Can you work these out from the model? Positions are in its coordinate system, mm. A direction names the side the tool comes from. Coordinates: 2 decimals unless noted, no trailing zeros. Order: outer loops, then holes, each group sorted by start corner. A loop starts at its lowest first (then second) coordinate and runs counter-clockwise, first axis right, second up.
```python
from build123d import *

# Parameters (mm, degrees)
SKETCH1_W           = 76.2
SKETCH1_H           = 25.4
SKETCH1_W_2         = 69.85
SKETCH1_H_2         = 19.05
BOSS_EXTRUDE1_DEPTH = 1016
SKETCH2_R           = 5.0419
CUT_EXTRUDE1_DEPTH  = 77.2
SKETCH3_R           = 3.3782
CUT_EXTRUDE2_DEPTH  = 26.4
SKETCH4_R           = 3.3782
CUT_EXTRUDE3_DEPTH  = 26.4


with BuildPart() as part:
    # Sketch1 → Boss-Extrude1 (new body)
    with BuildSketch(Plane(origin=(0, 0, 0), x_dir=(1, 0, 0), z_dir=(0, 1, 0))):
        with Locations((38.1, 12.7)):
            Rectangle(SKETCH1_W, SKETCH1_H)
        with Locations((38.1, 12.7)):
            Rectangle(SKETCH1_W_2, SKETCH1_H_2, mode=Mode.SUBTRACT)
    extrude(amount=BOSS_EXTRUDE1_DEPTH)

    # Sketch2 → Cut-Extrude1 (cut, through all)
    with BuildSketch(Plane(origin=(76.2, 0, 0), x_dir=(0, 0, -1), z_dir=(1, 0, 0))):
        with Locations((12.7, 293.6875)):
            Circle(SKETCH2_R)
        with Locations((12.7, 331.7875)):
            Circle(SKETCH2_R)
    cut_extrude1 = extrude(amount=-CUT_EXTRUDE1_DEPTH, mode=Mode.SUBTRACT)

    # Mirror1: Cut-Extrude1 across plane
    add(cut_extrude1.mirror(Plane(origin=(0, 508, 0), x_dir=(0, 0, 1), z_dir=(0, -1, 0))), mode=Mode.SUBTRACT)

    # Sketch3 → Cut-Extrude2 (cut, through all)
    with BuildSketch(Plane.XY):
        with Locations((15.875, 15.875)):
            Circle(SKETCH3_R)
        with Locations((15.875, 60.325)):
            Circle(SKETCH3_R)
        with Locations((60.325, 15.875)):
            Circle(SKETCH3_R)
        with Locations((60.325, 60.325)):
            Circle(SKETCH3_R)
    extrude(amount=-CUT_EXTRUDE2_DEPTH, mode=Mode.SUBTRACT)

    # Sketch4 → Cut-Extrude3 (cut, through all)
    with BuildSketch(Plane.XY):
        with Locations((50.8, 166.2938)):
            Circle(SKETCH4_R)
        with Locations((50.8, 656.0312)):
            Circle(SKETCH4_R)
    extrude(amount=-CUT_EXTRUDE3_DEPTH, mode=Mode.SUBTRACT)


solid = part.part
```
1. On a 3-axis mill with a long thin cutter (end or side, diameter ignored), from which of +Z, -Z, +X, -X, +Y, -Y can I reach the whole of each face in a straight line? I mean faces 1 (the flat face through (35, 0, -2)), 2 (the flat face through (38, 501, -22.225)). Say none if no direction works.
Completed:
face 1: +Z, -Z, +X, -X, -Y
face 2: +Y, -Y
2. Imagine slicing it at B-B on z = -12.7. Give the number of separate pieces and of enclosed holes in the cut face, then the cut area to 3 significant figures.
Completed:
separate pieces: 10
enclosed holes: 0
area: 6,200 mm2
3. Please list where these lines run through material, in increasing order: probe 1 along Y at (x, z) = (50.8, -1.55); probe 2 along Y at (x, z) = (74.15, -12.7); probe 3 along Z at (x, y) = (68.5, 612) (3 decimals).
Completed:
probe 1: y = 0 to 162.92, 169.67 to 652.65, 659.41 to 1016
probe 2: y = 0 to 288.65, 298.73 to 326.75, 336.83 to 679.17, 689.25 to 717.27, 727.35 to 1016
probe 3: z = -25.4 to -22.225, -3.175 to 0
4. Imagine slicing it at A-A on y = 369. Please give me the cut outline in (x, z) (3 decimals).
Completed:
outline: (0, -25.4) - (76.2, -25.4) - (76.2, 0) - (0, 0) - close; hole (3.175, -22.225) - (73.025, -22.225) - (73.025, -3.175) - (3.175, -3.175) - close
5. Thinking about a two-plate mould opening in Z: for faces 3 (the flat face through (38, 501, 0)), 4 (the flat face through (3.175, 501, -13)), 5 (the flat face through (0, 501, -13)), which applies, pulls with the +Z half, pulls with the -Z half, needs draft (parallel to the pull), parting line crosses it, or undercut?
Completed:
face 3: pulls with the +Z half
face 4: undercut
face 5: needs draft
